Check sheet for the modelled part. Datum: model origin and axes. Units: mm. A direction names the side the tool comes from. Round coordinates to 2 decimals unless told otherwise and drop trailing zeros. Loops run counter-clockwise (first coordinate to the right, second up) from the corner with the lowest first, then second, coordinate; pieces in that order, holes last. Notation, with made-up numbers: (52.25, 73.5) - (111.25, 73.5) arc R24 ccw to (111.25, 87.5) - close; hole circle Ø4 at (39.25, 42.5). An arc over 180 degrees is marked (long way). Put each result on its own line as item: value.
```python
from build123d import *

# Parameters (mm, degrees)
EXTRUDE015_DEPTH = 27.5
EXTRUDE_DEPTH    = 17


with BuildPart() as extrude015:
    # Sketch020 → Extrude015 (new body)
    with BuildSketch(Plane(origin=(-6, 0, 0), x_dir=(0, -1, 0), z_dir=(-1, 0, 0))):
        Polygon((19.5, -10.1), (19.5, -9.1), (5, -9.1), (4, -10.1), align=None)
    extrude(amount=EXTRUDE015_DEPTH)


with BuildPart() as cut006:
    # Sketch001 → Extrude (new body)
    with BuildSketch(Plane.XZ.offset(25)):
        with BuildLine():
            ThreePointArc((-7.6, 0), (-5.374012, -5.374012), (0, -7.6))
            Line((0, -7.6), (0, -9.6))
            Line((0, -9.6), (-34.6, -9.6))
            Line((-34.6, -9.6), (-34.6, -5.6))
            Line((-33.6, -5.6), (-34.6, -5.6))
            Line((-33.6, -6.6), (-33.6, -5.6))
            Line((-33.6, -6.6), (-9.6, -6.6))
            ThreePointArc((-9.6, -6.6), (-8.35, -5.35), (-9.6, -4.1))
            Line((-9.6, -4.1), (-21.6, -4.1))
            Line((-21.6, -4.1), (-21.6, -2.1))
            Line((-21.6, -2.1), (-11.7, -2.1))
            ThreePointArc((-11.7, -2.1), (-10.215076, -1.484924), (-9.6, 0))
            Line((-9.6, 0), (-7.6, 0))
        make_face()
    extrude(amount=-EXTRUDE_DEPTH)


with BuildPart() as cut006_1:
    # Extrude placement: moved
    add(cut006.part.moved(Location((0, 4.5, 0))))

    # Cut006: cut Extrude015
    add(extrude015.part, mode=Mode.SUBTRACT)


solid = cut006_1.part
```
Item 1: Section check A-A on x = -15. Enter the section's corners in (y, z).
Filled sheet:
outline: (-20.5, -9.6) - (-19.5, -9.6) - (-19.5, -9.1) - (-5, -9.1) - (-4.5, -9.6) - (-3.5, -9.6) - (-3.5, -6.6) - (-20.5, -6.6) - close; (-20.5, -4.1) - (-3.5, -4.1) - (-3.5, -2.1) - (-20.5, -2.1) - close
Item 2: Go/stop test with flat-tipped pins: pin 1 (1.5 mm diameter, centred on y = -6.5, z = -2, fed in from -X); pin 2 (0.8 mm diameter, centred on y = -16, z = -6, fed in from +X); pin 3 (3 mm diameter, centred on x = -18, y = -8, fed in from +Z). Record where each tip stops, or that it passes through.
Filled sheet:
pin 1: x = -21.6
pin 2: x = -4.1
pin 3: z = -2.1
Item 3: Thickness scan on line 1 (Z direction, x = -20, y = -14); line 2 (Z direction, x = -25, y = -8.5); line 3 (Z direction, x = -31.5, y = -4.75). Record the ranges inside material, lowest first. Write a range as from..to.
Filled sheet:
line 1: -9.1..-6.6, -4.1..-2.1
line 2: -9.1..-6.6
line 3: -9.35..-6.6
Item 4: Section check D-D on z = -5. Enter the section's corners in (x, y).
Filled sheet:
outline: (-8.4, -20.5) - (-5.72, -20.5) - (-5.72, -3.5) - (-8.4, -3.5) - close
Item 5: Release check for a two-part mould opening along X. For faces 5 (the cylindrical face through (-8.35, -12.12, -5.38)), 6 (the flat face through (-17, -20.5, -7)), 7 (the flat face through (-22, -12, -6.6)), 8 (the flat face through (0, -12, -9)) record: +X half, -X half, draft (parallel to the pull), parting line (faces both ways), or undercut.
Filled sheet:
face 5: undercut
face 6: draft
face 7: undercut
face 8: +X half
Item 6: Section check B-B on y = -16. Enter the section's corners in (x, z), then the cut area to 3 significant figures.
Filled sheet:
outline: (-34.6, -9.6) - (-33.5, -9.6) - (-33.5, -9.1) - (-6, -9.1) - (-6, -9.6) - (0, -9.6) - (0, -7.6) arc R7.6 cw to (-7.6, 0) - (-9.6, 0) arc R2.1 cw to (-11.7, -2.1) - (-21.6, -2.1) - (-21.6, -4.1) - (-9.6, -4.1) arc R1.25 cw to (-9.6, -6.6) - (-33.6, -6.6) - (-33.6, -5.6) - (-34.6, -5.6) - close
area: 132 mm²
Item 7: Tool access check on faces 1 (the flat face through (-17, -12, -2.1)), 2 (the flat face through (-33.6, -12, -6)), 3 (the flat face through (-20, -12, -9.1)), 4 (the flat face through (-16, -12, -4.1)). Record the directions out of +Z, -Z, +X, -X, +Y, -Y that give a thin tool (end or side, any length) a straight path to the whole face; none if there is none.
Filled sheet:
face 1: +Z, -X, +Y, -Y
face 2: +Z, +Y, -Y
face 3: -Z
face 4: -X, +Y, -Y
Item 8: Section check C-C on x = -26. Enter the section's corners in (y, z), then the cut area to 3 significant figures.
Filled sheet:
outline: (-20.5, -9.6) - (-19.5, -9.6) - (-19.5, -9.1) - (-5, -9.1) - (-4.5, -9.6) - (-3.5, -9.6) - (-3.5, -6.6) - (-20.5, -6.6) - close
area: 43.6 mm²
